Geometry check sheet. Reference: the model listing, model coordinates, mm. Face numbers are marked on the shaded views. A direction names the side the tool comes from. Round coordinates to 2 decimals unless told otherwise and drop trailing zeros. Order: outer loops, then holes, each group sorted by start corner. A loop starts at its lowest first (then second) coordinate and runs counter-clockwise, first axis right, second up. Notation, with made-up numbers: (14.5, 62) - (71.5, 62) arc R12 ccw to (71.5, 69) - close; hole circle Ø4 at (28, 47.5). An arc over 180 degrees is marked (long way). Write each question's results on one line, items separated by ' | '.
```python
from build123d import *

# Parameters (mm, degrees)
F0_W     = 80
F0_H     = 80
F1_DEPTH = 6
F2_W     = 60
F2_H     = 60
F3_DEPTH = 10
F4_R     = 1.5
F5_DEPTH = 8
F6_R     = 1.5
F7_DEPTH = 6


with BuildPart() as f1:
    # F0 (on Top) → F1 (new body)
    with BuildSketch(Plane.XY):
        Rectangle(F0_W, F0_H)
    extrude(amount=F1_DEPTH)

    # F2 (on face) → F3 (join)
    with BuildSketch(Plane.XY.offset(6)):
        Rectangle(F2_W, F2_H)
    extrude(amount=F3_DEPTH)

    # F4 (on face) → F5 (join)
    with BuildSketch(Plane.XY.offset(16)):
        with Locations((-27, -27)):
            Circle(F4_R)
        with Locations((27, -27)):
            Circle(F4_R)
        with Locations((27, 27)):
            Circle(F4_R)
        with Locations((-27, 27)):
            Circle(F4_R)
    extrude(amount=F5_DEPTH)

    # F6 (on face) → F7 (cut)
    with BuildSketch(Plane.XY.offset(6)):
        with Locations((-37, 37)):
            Circle(F6_R)
        with Locations((37, 37)):
            Circle(F6_R)
        with Locations((-37, -37)):
            Circle(F6_R)
        with Locations((37, -37)):
            Circle(F6_R)
    extrude(amount=-F7_DEPTH, mode=Mode.SUBTRACT)


solid = f1.part
```
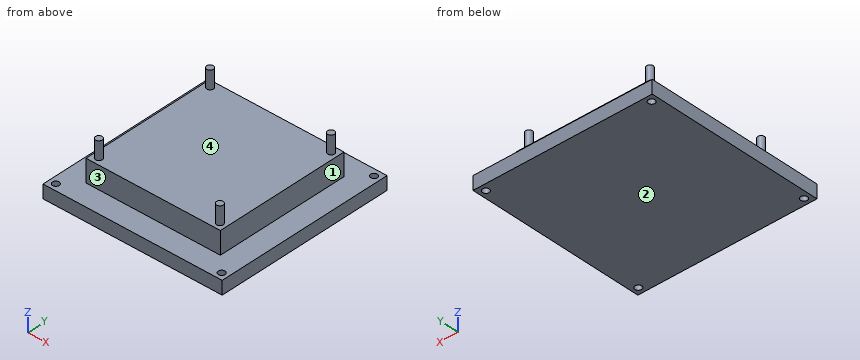
(1) Access from +Z, -Z, +X, -X, +Y, -Y to the whole of each face (thin tool, end or side, straight path). Record for the marked faces 1, 2, 3 and 4.
Answers follow:
face 1: +Z, +X, +Y, -Y | face 2: -Z, +X, -X, +Y, -Y | face 3: +Z, +X, -X, -Y | face 4: +Z
(2) Section check C-C (x = 27). Record the cut outline in (y, z).
Answers follow:
outline: (-40, 0) - (40, 0) - (40, 6) - (30, 6) - (30, 16) - (28.5, 16) - (28.5, 24) - (25.5, 24) - (25.5, 16) - (-25.5, 16) - (-25.5, 24) - (-28.5, 24) - (-28.5, 16) - (-30, 16) - (-30, 6) - (-40, 6) - close
(3) Section check A-A (x = -37). Record the cut outline in (y, z), then the cut area to 3 significant figures.
Answers follow:
outline: (-40, 0) - (-38.5, 0) - (-38.5, 6) - (-40, 6) - close; (-35.5, 0) - (35.5, 0) - (35.5, 6) - (-35.5, 6) - close; (38.5, 0) - (40, 0) - (40, 6) - (38.5, 6) - close | area: 444 mm²
(4) Depth check by flat-ended pin: pin 1 Ø3 at (y, z) = (13, 8.5) entering from -X; pin 2 Ø12 at (x, z) = (16.5, 11.5) entering from -Y; pin 3 Ø5 at (x, y) = (25.5, 2.5) entering from +Z; pin 4 Ø5 at (x, z) = (-12, 12) entering from +Y. Enter the tip coordinate at first touch or a pass-through.
Answers follow:
pin 1: x = -30 | pin 2: y = -40 | pin 3: z = 16 | pin 4: y = 30
(5) Material ranges on line 1 (Y direction, x = 37, z = 3.85); line 2 (X direction, y = -17, z = 15.75), recorded low to high.
Answers follow:
line 1: -40 to -38.5, -35.5 to 35.5, 38.5 to 40 | line 2: -30 to 30
(6) Section check D-D (z = 18.5). Record the cut outline in (x, y), then the cut area to 3 significant figures.
Answers follow:
outline: circle Ø3 at (-27, -27); circle Ø3 at (-27, 27); circle Ø3 at (27, -27); circle Ø3 at (27, 27) | area: 28.3 mm²
